```python
from build123d import *

# Parameters (mm, degrees)
F0_R     = 1.25
F0_R_2   = 1
F1_DEPTH = 20


# Not quite as in the source:
# - a fillet or chamfer that OpenCascade refuses, or shapes differently, is made with other operations: its cross-section is extruded or revolved along the edge and cut away or added


with BuildPart() as f1:
    # F0 (on Front) → F1 (new body)
    with BuildSketch(Plane.XZ):
        with Locations((-30.6629948318, 34.7370989621)):
            Circle(F0_R)
        with Locations((-30.6629948318, 34.7370989621)):
            Circle(F0_R_2, mode=Mode.SUBTRACT)
    extrude(amount=F1_DEPTH)

    # F2: fillet of radius 0.5 on 1 edges, made by hand

    # F2_s1 → F2_t2 (revolve, cut)
    with BuildSketch(Plane.XY.offset(34.7370989621)):
        with BuildLine():
            ThreePointArc((-29.4129948318, -19.5669872981), (-29.4799821299, -19.8169872981), (-29.6629948318, -20))
            Line((-29.6629948318, -20), (-29.4129948318, -20))
            Line((-29.4129948318, -20), (-29.4129948318, -19.5669872981))
        make_face()
    revolve(axis=Axis((-30.6629948318, -20, 34.7370989621), (0, -1, 0)), mode=Mode.SUBTRACT)

    # F3: fillet of radius 0.5 on 1 edges, made by hand

    # F3_s1 → F3_t2 (revolve, cut)
    with BuildSketch(Plane.XY.offset(34.7370989621)):
        with BuildLine():
            ThreePointArc((-29.4129948318, -0.4330127019), (-29.4799821299, -0.1830127019), (-29.6629948318, 0))
            Line((-29.6629948318, 0), (-29.4129948318, 0))
            Line((-29.4129948318, 0), (-29.4129948318, -0.4330127019))
        make_face()
    revolve(axis=Axis((-30.6629948318, 0, 34.7370989621), (0, -1, 0)), mode=Mode.SUBTRACT)


solid = f1.part
```
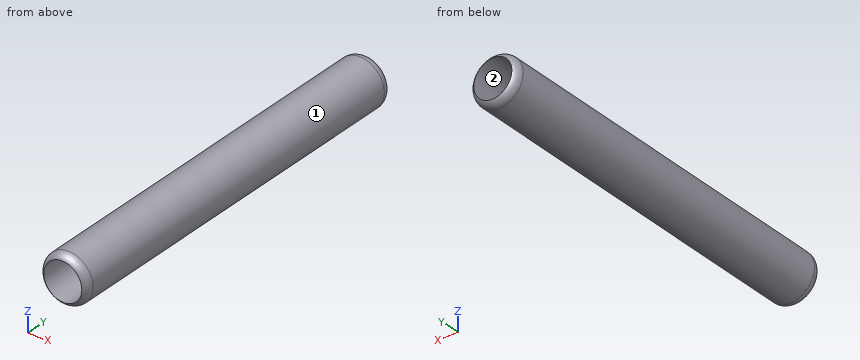
Verification items for the finished model (mm, model axes). Face numbers are marked on the shaded views. Coordinates: 2 decimals unless noted, no trailing zeros. Order: outer loops, then holes, each group sorted by start corner. A loop starts at its lowest first (then second) coordinate and runs counter-clockwise, first axis right, second up. Notation, with made-up numbers: (-3.5, 71.5) -> (1.5, 71.5) arc R24 cw to (1.5, 85.5) -> close; hole circle Ø5 at (-35, 61.25). An arc over 180 degrees is marked (long way). Put each result on its own line as item: value. Start each with the question number.
1) Cross-section at A-A (y = -15.5). Enter the section's corners in (x, z), plus the area to 3 significant figures.
2) Material ranges on L1, parallel to Z at x = -30.7, y = -1.5; L2, parallel to Z at x = -29.9, y = -14; L3, parallel to X at y = -15.25, z = 34.2, recorded low to high.
3) Go/stop test with a flat-tipped pin: pin 1 (1.5 mm diameter, centred on x = -31, y = -3, fed in from -Z). Record where the tip stops, or that it passes through.
4) Release check for a two-part mould opening along Z. For the marked faces 1 and 2 record: pulls with the +Z half, pulls with the -Z half, needs draft (parallel to the pull), parting line crosses it, or undercut.
Geometry check:
1. outline: circle Ø2.5 at (-30.66, 34.74); hole circle Ø2 at (-30.66, 34.74)
1. area: 1.77 mm^2
2. L1: z = 33.49 to 33.74, 35.74 to 35.99
2. L2: z = 33.75 to 34.09, 35.38 to 35.73
2. L3: x = -31.79 to -31.51, -29.82 to -29.53
3. pin 1: stops at z = 33.49
4. face 1: parting line crosses it
4. face 2: undercut
